```python
from build123d import *

# Parameters (mm, degrees)
BOSS_EXTRUDE1_DEPTH = 35.56
FILLET1_R           = 12.7


with BuildPart() as part:
    # Sketch1 → Boss-Extrude1 (new body)
    with BuildSketch(Plane.XY):
        with BuildLine():
            Line((85.09, 0), (85.09, 21.59))
            Line((85.09, 21.59), (2.54, 21.59))
            Line((2.54, 21.59), (0, 0))
            Line((0, 0), (17.78, 0))
            ThreePointArc((17.78, 0), (20.32, 2.54), (22.86, 0))
            Line((22.86, 0), (62.23, 0))
            ThreePointArc((62.23, 0), (64.77, 2.54), (67.31, 0))
            Line((67.31, 0), (85.09, 0))
        make_face()
    extrude(amount=BOSS_EXTRUDE1_DEPTH)

    # Fillet1
    fillet1_edges = [part.edges().sort_by_distance(p)[0] for p in [
        (2.54, 21.59, 17.78),
    ]]
    fillet(fillet1_edges, radius=FILLET1_R)


solid = part.part
```
Check sheet for the modelled part. Datum: model origin and axes. Units: mm. Round coordinates to 2 decimals unless told otherwise and drop trailing zeros. Order: outer loops, then holes, each group sorted by start corner. A loop starts at its lowest first (then second) coordinate and runs counter-clockwise, first axis right, second up. Notation, with made-up numbers: (46.25, -34) - (85.25, -34) arc R18 ccw to (85.25, -5) - close; hole circle Ø2 at (-27, 11). An arc over 180 degrees is marked (long way). Answer as CSV lines item,"result". Start each with the question number.
1) Depth check by flat-ended pin: pin 1 (12 mm diameter, centred on x = 17, z = 14, fed in from -Y); pin 2 (2 mm diameter, centred on y = 8.5, z = 18, fed in from -X); pin 3 (4 mm diameter, centred on y = 13.5, z = 22.5, fed in from -X). Enter the tip coordinate at first touch or a pass-through.
2) Section check C-C (y = 13.5). Record the cut outline in (x, z), then the cut area to 3 significant figures.
3) Scan lines: probe 1 along X at (y, z) = (1.75, 28.5); probe 2 along X at (y, z) = (1.5, 7.5); probe 3 along X at (y, z) = (11.25, 32). Record each from-to range of solid material in increasing order.
4) Section check A-A (z = 31). Record the cut outline in (x, y).
5) Section check B-B (x = 64.77). Record the cut outline in (y, z).
6) Draft check along X on faces 1 (the face through (42, 0, 18)), 2 (the face through (20.26, 2.54, 17.53)), 3 (the face through (64.71, 2.54, 17.53)), 4 (the face through (0.62, 5.26, 17.53)). Enter one of: +X half, -X half, draft (parallel to the pull), parting line (faces both ways), or undercut.
Determined:
1,pin 1,"y = 0"
1,pin 2,"x = 0.88"
1,pin 3,"x = 1.4"
2,outline,"(2, 0) - (85.09, 0) - (85.09, 35.56) - (2, 35.56) - close"
2,area,"2,950 mm^2"
3,probe 1,"0.21 to 18.48, 22.16 to 62.93, 66.61 to 85.09"
3,probe 2,"0.18 to 18.27, 22.37 to 62.72, 66.82 to 85.09"
3,probe 3,"1.35 to 85.09"
4,outline,"(0, 0) - (17.78, 0) arc R2.54 cw to (22.86, 0) - (62.23, 0) arc R2.54 cw to (67.31, 0) - (85.09, 0) - (85.09, 21.59) - (13.83, 21.59) arc R12.7 ccw to (1.22, 10.37) - close"
5,outline,"(2.54, 0) - (21.59, 0) - (21.59, 35.56) - (2.54, 35.56) - close"
6,face 1,"draft"
6,face 2,"undercut"
6,face 3,"undercut"
6,face 4,"-X half"
